Check sheet for the drawn part. Datum: minimum x, y, z corner. Units: mm. Round coordinates to 2 decimals unless told otherwise and drop trailing zeros. Write each loop counter-clockwise with the first axis right and the second up, starting at its lowest first coordinate (ties: lowest second). Pieces come first, ordered by that corner, then holes.
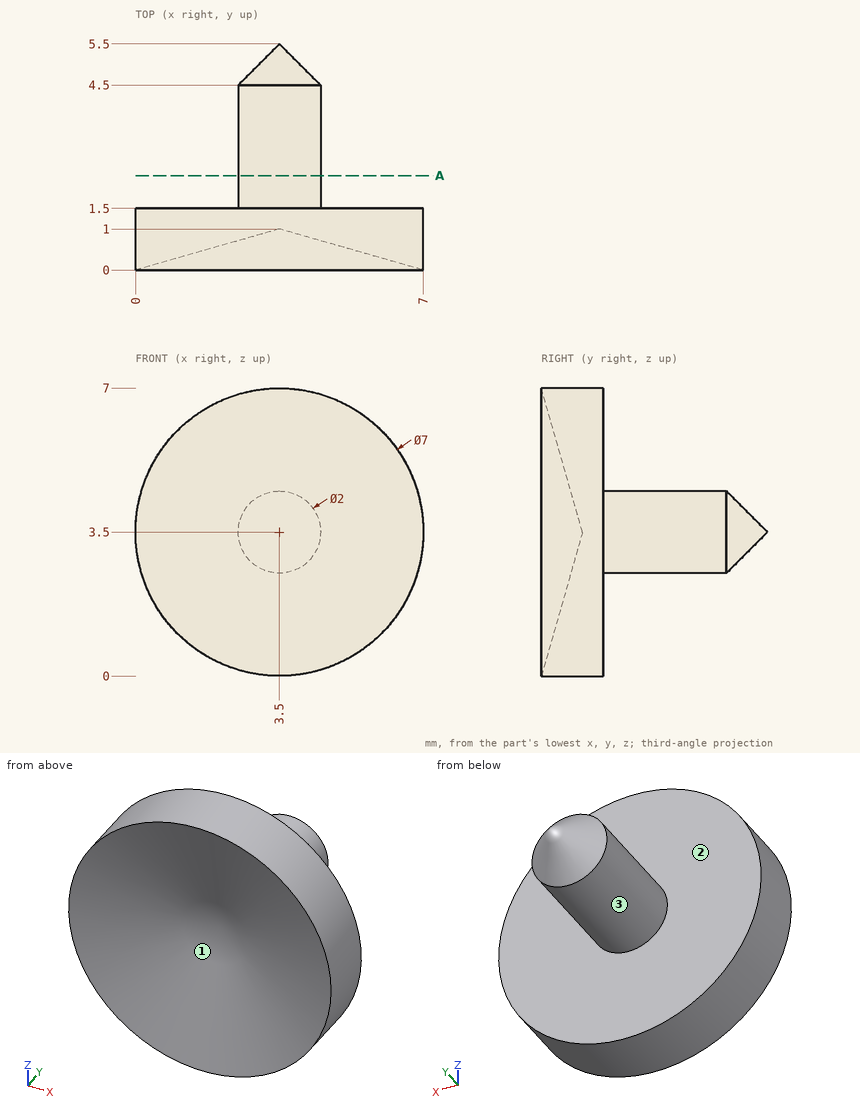
Q1. Release check for a two-part mould opening along Z. For the marked faces 1, 2 and 3 record: released by +Z, released by -Z, zero draft, split by the parting line, or undercut.
Recorded:
face 1: undercut
face 2: zero draft
face 3: split by the parting line
Q2. Sectioned sample at A-A (y = 2.3). Enter the section's corners in (x, z).
Recorded:
outline: circle Ø2 at (3.5, 3.5)
Q3. Depth check by flat-ended pin: P1, Ø1.5, axis at x = 4, y = 4, coming from the -Z side; P2, Ø1, axis at x = 1, z = 6, coming from the -Y side. Enter the tip coordinate at first touch or a pass-through.
Recorded:
P1: stops at z = 2.5
P2: stops at y = 0
Q4. Material ranges on line 1 along Y through (x, z) = (1, 4.5); line 2 along X through (y, z) = (1.2, 5.25); line 3 along X through (y, z) = (4.9, 3.75), recorded low to high.
Recorded:
line 1: y = 0.23 to 1.5
line 2: x = 0.47 to 6.53
line 3: x = 2.95 to 4.05
